from build123d import *

# Parameters (mm, degrees)
SKETCH_1_W          = 86
SKETCH_1_H          = 20
EXTRUDE_1_DEPTH     = 3.5
SKETCH_2_R          = 3.25
CUT_EXTRUDE_1_DEPTH = 3.5
SKETCH_3_W          = 3
SKETCH_3_H          = 20
EXTRUDE_2_DEPTH     = 30
FILLET_1_R          = 5
FILLET_2_R          = 5
SKETCH_4_R          = 1.65
CUT_EXTRUDE_2_DEPTH = 91
FILLET_3_R          = 5
SKETCH_6_R          = 1.65
CUT_EXTRUDE_3_DEPTH = 2
SKETCH_7_R          = 1.65
CUT_EXTRUDE_4_DEPTH = 1
SKETCH_8_W          = 80.307081952
SKETCH_8_H          = 1.75
EXTRUDE_3_DEPTH     = 3


with BuildPart() as part:
    # 草图1 → 凸台-拉伸1 (new body)
    with BuildSketch(Plane(origin=(0, 0, 0), x_dir=(1, 0, 0), z_dir=(0, 1, 0))):
        Rectangle(SKETCH_1_W, SKETCH_1_H)
    extrude(amount=EXTRUDE_1_DEPTH)

    # 草图2 → 切除-拉伸1 (cut)
    with BuildSketch(Plane(origin=(0, 3.5, 0), x_dir=(1, 0, 0), z_dir=(0, 1, 0))):
        with Locations(Location((0, 0, 0), (0, 0, 270))):
            Circle(SKETCH_2_R)
    extrude(amount=-CUT_EXTRUDE_1_DEPTH, mode=Mode.SUBTRACT)

    # 草图3 → 凸台-拉伸2 (add)
    with BuildSketch(Plane(origin=(0, 3.5, 0), x_dir=(1, 0, 0), z_dir=(0, 1, 0))):
        with Locations((41.5, 0)):
            Rectangle(SKETCH_3_W, SKETCH_3_H)
        with Locations((-41.5, 0)):
            Rectangle(SKETCH_3_W, SKETCH_3_H)
    extrude(amount=EXTRUDE_2_DEPTH)

    # 圆角1
    fillet_1_edges = [part.edges().sort_by_distance(p)[0] for p in [
        (-40, 3.5, 0),
    ]]
    fillet(fillet_1_edges, radius=FILLET_1_R)

    # 圆角2
    fillet_2_edges = [part.edges().sort_by_distance(p)[0] for p in [
        (40, 3.5, 0),
    ]]
    fillet(fillet_2_edges, radius=FILLET_2_R)

    # 草图4 → 切除-拉伸2 (cut)
    with BuildSketch(Plane.ZY.offset(43)):
        with Locations((0, 28.5)):
            Circle(SKETCH_4_R)
    extrude(amount=-CUT_EXTRUDE_2_DEPTH, mode=Mode.SUBTRACT)

    # 圆角3
    fillet_3_edges = [part.edges().sort_by_distance(p)[0] for p in [
        (41.5, 33.5, -10),
        (41.5, 33.5, 10),
        (-41.5, 33.5, 10),
        (-41.5, 33.5, -10),
    ]]
    fillet(fillet_3_edges, radius=FILLET_3_R)

    # 草图6 → 切除-拉伸3 (cut)
    with BuildSketch(Plane.ZY.offset(43)):
        with BuildLine():
            Line((2.240090483, 12.2890625), (3.733484138, 28.1484375))
            ThreePointArc((3.733484138, 28.1484375), (0, 32.25), (-3.733484138, 28.1484375))
            Line((-3.733484138, 28.1484375), (-2.240090483, 12.2890625))
            ThreePointArc((-2.240090483, 12.2890625), (0, 10.25), (2.240090483, 12.2890625))
        make_face()
        with Locations((0, 28.5)):
            Circle(SKETCH_6_R, mode=Mode.SUBTRACT)
    extrude(amount=-CUT_EXTRUDE_3_DEPTH, mode=Mode.SUBTRACT)

    # 草图7 → 切除-拉伸4 (cut)
    # profile 1 of 3: a face of its own
    with BuildSketch(Plane.ZY.offset(41)):
        with BuildLine():
            ThreePointArc((3.75, 28.5), (-0.175975116, 32.245868759), (-3.733484138, 28.1484375))
            ThreePointArc((-3.733484138, 28.1484375), (0, 24.75), (3.733484138, 28.1484375))
            ThreePointArc((3.733484138, 28.1484375), (3.745868759, 28.324024884), (3.75, 28.5))
        make_face()
        with Locations((0, 28.5)):
            Circle(SKETCH_7_R, mode=Mode.SUBTRACT)
    # profile 2 of 3: a face of its own
    with BuildSketch(Plane.ZY.offset(41)):
        with BuildLine():
            Line((-3.733484138, 28.1484375), (-3.199423337, 22.476878304))
            Line((-3.199423337, 22.476878304), (3.199423337, 22.476878304))
            Line((3.199423337, 22.476878304), (3.733484138, 28.1484375))
            ThreePointArc((3.733484138, 28.1484375), (0, 24.75), (-3.733484138, 28.1484375))
        make_face()
    # profile 3 of 3: a face of its own
    with BuildSketch(Plane.ZY.offset(41)):
        with BuildLine():
            Line((-1, 20.5), (-1, 12.5))
            ThreePointArc((-1, 12.5), (0, 11.5), (1, 12.5))
            Line((1, 12.5), (1, 20.5))
            ThreePointArc((1, 20.5), (0, 21.5), (-1, 20.5))
        make_face()
    extrude(amount=-CUT_EXTRUDE_4_DEPTH, mode=Mode.SUBTRACT)

    # 草图8 → 凸台-拉伸3 (add)
    with BuildSketch(Plane(origin=(0, 3.5, 0), x_dir=(1, 0, 0), z_dir=(0, 1, 0))):
        with Locations((0.153540976, 9.125)):
            Rectangle(SKETCH_8_W, SKETCH_8_H)
    extrude(amount=EXTRUDE_3_DEPTH)


solid = part.part
The model under review builds one solid part; all positions refer to its coordinate system, in mm. A direction names the side the tool comes from. Give positions to 0.01 mm unless a question says otherwise; leave off trailing zeros. Order: outer loops, then holes, each group sorted by start corner. A loop starts at its lowest first (then second) coordinate and runs counter-clockwise, first axis right, second up. Notation, with made-up numbers: M -9,29 L -5,29 A19 cw -5,51 Z; hole C 63,-25.75 d11. An arc over 180 degrees is marked long. Use one line per item in the form item = value. Start each with the question number.
Item 1: Insertion check: pin 1 Ø5 at (x, z) = (-2, 5) entering from +Y; pin 2 Ø0.9 at (x, z) = (-19.5, -9.5) entering from +Y. Each pin has a flat end and moves straight along its axis. Give the tip position at first contact, or say it passes through.
Item 2: The part is to be moulded in two halves that separate along Z. For faces 1 (the cylindrical face through (-38.57, 5, -0.14)), 2 (the cylindrical face through (41.479, 30.136, -0.215)), 3 (the flat face through (0, 2, 10)), say which applies: pulls with the +Z half, pulls with the -Z half, needs draft (parallel to the pull), parting line crosses it, or undercut.
Item 3: We need section B-B on x = 0. Give the boundary of the cut face in (y, z).
Item 4: We need section C-C on y = 14.5. Give the boundary of the cut face in (x, z), plus the area to 3 significant figures.
Item 5: We need section A-A on z = 0. Give the boundary of the cut face in (x, y).
Item 6: To check wall thickness, follow line 1 along X through (y, z) = (27, 6.25); line 2 along Z through (x, y) = (-41, 28); line 3 along X through (y, z) = (0.75, 0). State the ranges of each line that lie inside material, in increasing order. Write a range as from..to.
Item 7: For faces 4 (the cylindrical face through (41.52, 32, 8.57)), 5 (the flat face through (0, 3.5, 5)), 6 (the cylindrical face through (-42.01, 10.25, -0.05)), 7 (the flat face through (40, 21, 0)), 8 (the flat face through (0, 5, -10)), list the 3-axis set-ups (+Z, -Z, +X, -X, +Y, -Y) from which the entire face can be reached by the end or side of a thin tool; tool diameter is ignored.
Item 8: We need section D-D on z = 6. Give the boundary of the cut face in (x, y), plus the area to 3 significant figures.
Completed:
q1.pin_1 = 3.5
q1.pin_2 = 6.5
q2.face_1 = needs draft
q2.face_2 = undercut
q2.face_3 = pulls with the +Z half
q3.outline = M 0,-10 L 6.5,-10 L 6.5,-8.25 L 3.5,-8.25 L 3.5,-3.25 L 0,-3.25 Z; M 0,3.25 L 3.5,3.25 L 3.5,10 L 0,10 Z
q4.outline = M -43,-10 L -40,-10 L -40,-1 L -41,-1 L -41,-2.45 L -43,-2.45 Z; M -43,2.45 L -41,2.45 L -41,1 L -40,1 L -40,10 L -43,10 Z; M 40,-10 L 43,-10 L 43,10 L 40,10 Z
q4.area = 108 mm²
q5.outline = M -43,0 L -3.25,0 L -3.25,3.5 L -35,3.5 A5 cw -40,8.5 L -40,11.5 L -41,11.5 L -41,10.25 L -43,10.25 Z; M -43,32.25 L -40,32.25 L -40,33.5 L -43,33.5 Z; M -41,21.5 L -40,21.5 L -40,22.48 L -41,22.48 Z; M 3.25,0 L 43,0 L 43,26.85 L 40,26.85 L 40,8.5 A5 cw 35,3.5 L 3.25,3.5 Z; M 40,30.15 L 43,30.15 L 43,33.5 L 40,33.5 Z
q6.line_1 = -43..-40, 40..43
q6.line_2 = -10..-3.72, 3.72..10
q6.line_3 = -43..-3.25, 3.25..43
q7.face_4 = +Z, +X, -X, +Y
q7.face_5 = +Z, +Y
q7.face_6 = -X
q7.face_7 = +Z, -Z, +Y
q7.face_8 = -Z, +X, -X, +Y, -Y
q8.outline = M -43,0 L 43,0 L 43,33.4 L 40,33.4 L 40,8.5 A5 cw 35,3.5 L -35,3.5 A5 cw -40,8.5 L -40,33.4 L -43,33.4 Z
q8.area = 491 mm²
